from build123d import *

# Parameters (mm, degrees)
F0_R      = 26.9875
F1_DEPTH  = 133.35
F2_R      = 22.225
F3_DEPTH  = 9.525
F4_R      = 26.9875
F5_DEPTH  = 9.525
F6_SIZE   = 1.5875
F9_DEPTH  = 9.525
F10_R     = 34.925
F11_DEPTH = 25.4
F12_DEPTH = 12.7


with BuildPart() as f1:
    # F0 (on Top) → F1 (new body)
    with BuildSketch(Plane.XY):
        Circle(F0_R)
    extrude(amount=F1_DEPTH)

    # F2 (on face) → F3 (join)
    with BuildSketch(Plane.XY.offset(133.35)):
        Circle(F2_R)
    extrude(amount=F3_DEPTH)

    # F4 (on face) → F5 (join)
    with BuildSketch(Plane.XY.offset(142.875)):
        Circle(F4_R)
    extrude(amount=F5_DEPTH)

    # F6
    f6_edges = [f1.edges().sort_by_distance(p)[0] for p in [
        (-26.9875, 0, 152.4),
    ]]
    chamfer(f6_edges, length=F6_SIZE)

    # F8 (on offset) → F9 (cut)
    with BuildSketch(Plane.YZ.offset(30.1625)):
        with BuildLine():
            Line((6.35, 63.4389315911), (6.35, 152.5463323689))
            Line((6.35, 152.5463323689), (-6.35, 152.5463323689))
            Line((-6.35, 152.5463323689), (-6.35, 63.4389315911))
            ThreePointArc((-6.35, 63.4389315911), (0, 57.0889315911), (6.35, 63.4389315911))
        make_face()
    extrude(amount=-F9_DEPTH, mode=Mode.SUBTRACT)

    # F10 (on face) → F11 (join)
    with BuildSketch(Plane(origin=(0, 0, 0), x_dir=(1, 0, 0), z_dir=(0, 0, -1))):
        Circle(F10_R)
    extrude(amount=-F11_DEPTH)

    # F12 (add): a face of the model
    f12_faces = [f1.faces().sort_by_distance(p)[0] for p in [
        (-33.9371718267, 0, 25.4),
    ]]
    extrude(f12_faces, amount=F12_DEPTH)


solid = f1.part
Can you work these out from the model? Positions are in its coordinate system, mm. A direction names the side the tool comes from. Coordinates: 2 decimals unless noted, no trailing zeros. Loops run counter-clockwise (first coordinate to the right, second up) from the corner with the lowest first, then second, coordinate; pieces in that order, holes last. Notation, with made-up numbers: (79, 66.5) - (92, 66.5) arc R18 cw to (92, 76.5) - close; hole circle Ø11 at (78, 51). An arc over 180 degrees is marked (long way). Answer as a JSON object with one key per item and string values. Group by question number.
Item 1: If we section it at C-C (z = 19.5): List the corners of the cut face in (x, y) for me (3 decimals), plus the area to 3 significant figures.
Item 2: For pin 1 (14 mm diameter, centred on y = -1, z = 88, fed in from +X); pin 2 (3 mm diameter, centred on y = 11, z = 59.5, fed in from -X); pin 3 (12 mm diameter, centred on y = -11.5, z = 98, fed in from -X), each with a flat end and sliding along its axis, tell me the tip position at first contact or that it passes through.
Item 3: On a 3-axis mill with a long thin cutter (end or side, diameter ignored), from which of +Z, -Z, +X, -X, +Y, -Y can I reach the whole of each face in a straight line? I mean faces 4 (the face through (-22.2, 4.1, 133.35)), 5 (the face through (23.86, -0.14, 57.09)), 6 (the face through (-27.715, 21.251, 18.783)), 7 (the face through (18, 21, 38.1)), 8 (the face through (-1, 0, 152.4)). Say none if no direction works.
Item 4: If we mould it in two halves opening along Z, with no side actions, what happens to faces 1 (the face through (20.638, 0, 105)), 2 (the face through (0, 0, 0)), 3 (the face through (-22.2, 4.1, 142.875))? For each: released by +Z, released by -Z, zero draft, split by the parting line, or undercut.
Item 5: If I drill on L1, parallel to Z at x = -15, y = 18 (3 decimals); L2, parallel to Z at x = -31, y = 1; L3, parallel to Z at x = 24, y = -11 (3 decimals), over which ranges is the centre line in solid material (lowest first)? Write a range as from..to.
Returned:
{
 "1": {"outline": "circle Ø69.85 at (0, 0)", "area": "3,830 mm²"},
 "2": {"pin 1": "stops at x = 26.23", "pin 2": "stops at x = -25.26", "pin 3": "stops at x = -26.42"},
 "3": {"face 4": "none", "face 5": "+Z, +X", "face 6": "+Z, -Z", "face 7": "+Z", "face 8": "+Z, +X, -X, +Y, -Y"},
 "4": {"face 1": "zero draft", "face 2": "released by -Z", "face 3": "undercut"},
 "5": {"L1": "z = 0..133.35, 142.875..152.4", "L2": "z = 0..38.1", "L3": "z = 0..133.35, 142.875..151.399"}
}
